```python
from build123d import *

# Parameters (mm, degrees)
BOSS_EXTRUDE1_DEPTH = 20
HOLE1_D             = 38
HOLE1_DEPTH         = 100
HOLE1_CBORE_D       = 54
HOLE1_CBORE_DEPTH   = 20
HOLE1_TIP           = 11.416351762
SKETCH4_R           = 19
BOSS_EXTRUDE2_DEPTH = 15
SKETCH5_R           = 5
BOSS_EXTRUDE3_DEPTH = 5


with BuildPart() as part:
    # Sketch1 → Boss-Extrude1 (new, symmetric)
    with BuildSketch(Plane(origin=(0, 0, 0), x_dir=(0, 0, -1), z_dir=(1, 0, 0))):
        Polygon((-38, 0), (-38, 64), (-44, 64), (-44, 69), (-30, 100), (30, 100), (44, 69), (44, 64), (38, 64), (38, 0), (18, 0), (18, 20), (-18, 20), (-18, 0), align=None)
    extrude(amount=BOSS_EXTRUDE1_DEPTH, both=True)

    # Hole1
    with Locations(Plane(origin=(20, 0, 0), x_dir=(0, 0, -1), z_dir=(1, 0, 0))):
        with Locations((0, 100)):
            CounterBoreHole(HOLE1_D / 2, HOLE1_CBORE_D / 2, HOLE1_CBORE_DEPTH, depth=HOLE1_DEPTH)
            with Locations((0, 0, -(HOLE1_DEPTH + HOLE1_TIP / 2))):  # 118° drill point
                Cone(0, HOLE1_D / 2, HOLE1_TIP, mode=Mode.SUBTRACT)

    # Sketch4 → Boss-Extrude2 (add)
    with BuildSketch(Plane.ZY.offset(20)):
        with Locations((0, 100)):
            Circle(SKETCH4_R)
    extrude(amount=-BOSS_EXTRUDE2_DEPTH)

    # Sketch5 → Boss-Extrude3 (add)
    with BuildSketch(Plane(origin=(0, 69, 0), x_dir=(1, 0, 0), z_dir=(0, 1, 0))):
        with BuildLine():
            Line((-10, 63), (-10, 44))
            Line((-10, 44), (10, 44))
            Line((10, 44), (10, 63))
            ThreePointArc((10, 63), (0, 73), (-10, 63))
        make_face()
        with Locations(Location((0, 63, 0), (0, 0, 270))):
            Circle(SKETCH5_R, mode=Mode.SUBTRACT)
    boss_extrude3 = extrude(amount=-BOSS_EXTRUDE3_DEPTH)

    # Mirror1: Boss-Extrude3 across plane
    add(boss_extrude3.mirror(Plane.XY))


solid = part.part
```
The listing builds one solid part. Answer for the finished solid, in the listing's coordinates (mm). A direction names the side the tool comes from. Give positions to 0.01 mm unless a question says otherwise; leave off trailing zeros. Order: outer loops, then holes, each group sorted by start corner. A loop starts at its lowest first (then second) coordinate and runs counter-clockwise, first axis right, second up.
Item 1: The part is cut by section B-B, the plane y = 67. Give the vertices of the cut face in (x, z).
From the geometry:
outline: (-20, -44) - (-10, -44) - (-10, -63) arc R10 ccw to (10, -63) - (10, -44) - (20, -44) - (20, 44) - (10, 44) - (10, 63) arc R10 ccw to (-10, 63) - (-10, 44) - (-20, 44) - close; hole circle Ø10 at (0, -63); hole circle Ø10 at (0, 63)
Item 2: The part is cut by section C-C, the plane z = 56. Give the vertices of the cut face in (x, y).
From the geometry:
outline: (-10, 64) - (10, 64) - (10, 69) - (-10, 69) - close
Item 3: Find the intervals of material crossed by probe 1 along X at (y, z) = (66.4, -63); probe 2 along X at (y, z) = (101, 4); probe 3 along Z at (x, y) = (18, 86.5), in increasing order.
From the geometry:
probe 1: x = -10 to -5, 5 to 10
probe 2: x = -20 to -5
probe 3: z = -36.1 to -23.38, 23.38 to 36.1
Item 4: Which of the six approach directions +Z, -Z, +X, -X, +Y, -Y give full straight-line access (tool end or side, diameter ignored) to faces 1 (the face through (0, 20, 0)), 2 (the face through (0, 69, 55)), 3 (the face through (-15, 67, -44)), 4 (the face through (10, 67, 53)), 5 (the face through (0, 69, -55))?
From the geometry:
face 1: +X, -X, -Y
face 2: +Z, +X, -X, +Y
face 3: -Z, -X, +Y, -Y
face 4: +Z, +X, +Y, -Y
face 5: -Z, +X, -X, +Y
Item 5: Given pin 1 Ø1.5 at (x, y) = (-13.5, 67) entering from -Z; pin 2 Ø6 at (x, y) = (-8.5, 8) entering from +Z; pin 3 Ø10 at (x, z) = (13.5, 46) entering from +Y; pin 4 Ø9 at (x, z) = (0, 63) entering from -Y, each flat-ended and moving along its own axis, determine where each tip first touches the part or whether it passes through.
From the geometry:
pin 1: stops at z = -44
pin 2: stops at z = 38
pin 3: stops at y = 75.64
pin 4: passes through
Item 6: The part is cut by section A-A, the plane x = 14. Give the vertices of the cut face in (y, z), and give its area (3 significant figures).
From the geometry:
outline: (0, -38) - (64, -38) - (64, -44) - (69, -44) - (100, -30) - (100, -27) arc R27 cw to (100, 27) - (100, 30) - (69, 44) - (64, 44) - (64, 38) - (0, 38) - (0, 18) - (20, 18) - (20, -18) - (0, -18) - close
area: 5,730 mm2
Item 7: For a pull along Z with two mould halves and no side action, classify faces 6 (the face through (0, 80.7, 0.4)), 7 (the face through (0, 0, 28)), 8 (the face through (15, 67, -44)) as pulls with the +Z half, pulls with the -Z half, needs draft (parallel to the pull), parting line crosses it, or undercut.
From the geometry:
face 6: undercut
face 7: needs draft
face 8: pulls with the -Z half
Item 8: The part is cut by section D-D, the plane y = 84. Give the vertices of the cut face in (x, z), and give its area (3 significant figures).
From the geometry:
outline: (-20, -37.23) - (20, -37.23) - (20, -21.75) - (0, -21.75) - (0, -10.25) - (-5, -10.25) - (-5, 10.25) - (0, 10.25) - (0, 21.75) - (20, 21.75) - (20, 37.23) - (-20, 37.23) - close
area: 2,010 mm2
